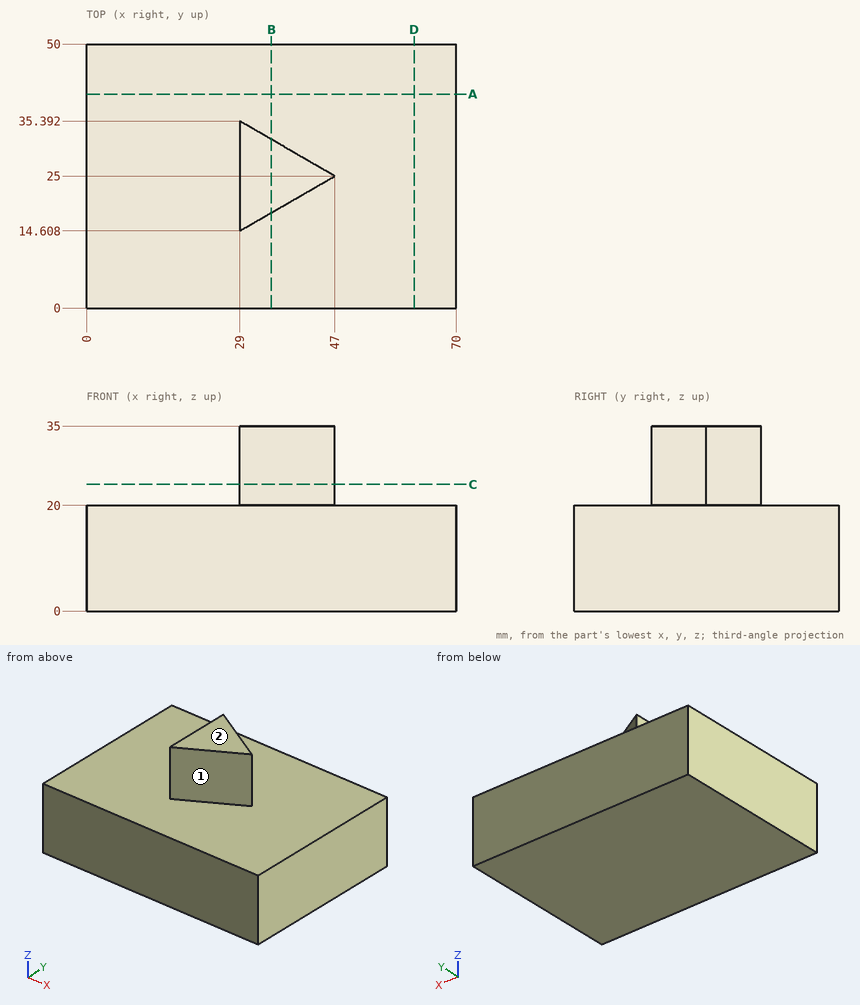
Could you check a few things on this drawing? It's one solid part, dimensions in mm from its lowest x, y, z. A direction names the side the tool comes from. Give positions to 0.01 mm unless a question says otherwise; leave off trailing zeros. Loops run counter-clockwise (first coordinate to the right, second up) from the corner with the lowest first, then second, coordinate; pieces in that order, holes last. Notation, with made-up numbers: (14, -12) -> (29, -12) arc R12 cw to (29, -4) -> close; hole circle Ø11 at (-35, 64). An arc over 180 degrees is marked (long way). Use one line per item in the form item = value. Start each with the question number.
1) Imagine slicing it at D-D (x = 62). Please give me the cut outline in (y, z), then the cut area to 3 significant figures.
2) Imagine slicing it at A-A (y = 40.5). Please give me the cut outline in (x, z).
3) Please list where these lines run through material, in increasing order: line 1 along Z through (x, y) = (58, 20.5); line 2 along Y through (x, z) = (36, 32.5); line 3 along X through (y, z) = (35, 26).
4) For P1, Ø6, axis at y = 7.5, z = 12, coming from the -X side; P2, Ø6, axis at x = 56.5, y = 12.5, coming from the +Z side; P3, Ø7.5, axis at y = 30, z = 28, coming from the -X side, each with a flat end and sliding along its axis, tell me the tip position at first contact or that it passes through.
5) Imagine slicing it at B-B (x = 35). Please give me the cut outline in (y, z).
6) Imagine slicing it at C-C (z = 24). Please give me the cut outline in (x, y), then the cut area to 3 significant figures.
7) Which directions (+Z, -Z, +X, -X, +Y, -Y) give clear straight access to the entire face, cutting with the end or side of a thin tool? Please do the marked faces 1 and 2.
Check values:
q1.outline = (0, 0) -> (50, 0) -> (50, 20) -> (0, 20) -> close
q1.area = 1,000 mm^2
q2.outline = (0, 0) -> (70, 0) -> (70, 20) -> (0, 20) -> close
q3.line_1 = 0 to 20
q3.line_2 = 18.65 to 31.35
q3.line_3 = 29 to 29.68
q4.P1 = 0
q4.P2 = 20
q4.P3 = 29
q5.outline = (0, 0) -> (50, 0) -> (50, 20) -> (31.93, 20) -> (31.93, 35) -> (18.07, 35) -> (18.07, 20) -> (0, 20) -> close
q6.outline = (29, 14.61) -> (47, 25) -> (29, 35.39) -> close
q6.area = 187 mm^2
q7.face_1 = +Z, +X, -Y
q7.face_2 = +Z, +X, -X, +Y, -Y
